Verification items for the finished model (mm, model axes). Face numbers are marked on the shaded views. A direction names the side the tool comes from. Coordinates: 2 decimals unless noted, no trailing zeros. Write each loop counter-clockwise with the first axis right and the second up, starting at its lowest first coordinate (ties: lowest second). Pieces come first, ordered by that corner, then holes. Notation, with made-up numbers: (31.5, 89.5) -> (81.5, 89.5) arc R17 ccw to (81.5, 100.5) -> close; hole circle Ø8 at (27, 55.5). An arc over 180 degrees is marked (long way). Use a Markdown table: item, result. Add a question column.
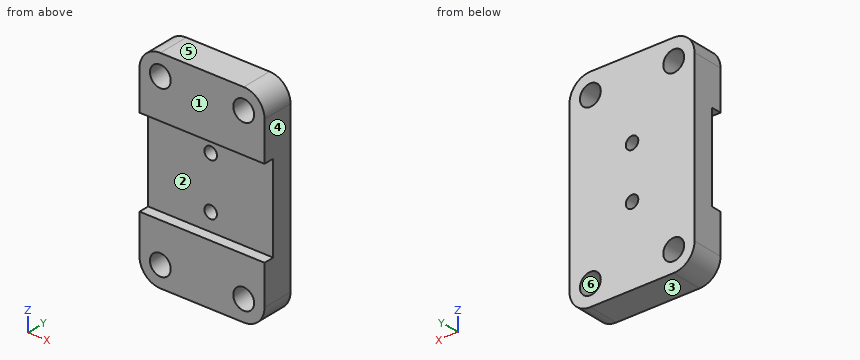
Autodesk Inventor part; units mm, degrees
ref_plane "YZ Plane" through (0, 0, 0) normal (1, 0, 0) x (0, 1, 0)
ref_plane "XZ Plane" through (0, 0, 0) normal (0, 1, 0) x (-1, 0, 0)
ref_plane "XY Plane" through (0, 0, 0) normal (0, 0, 1) x (1, 0, 0)
sketch "Sketch1" plane through (0, 0, 0) normal (0, 1, 0) x (-1, 0, 0)
  line L0 (30, 50) -> (-30, 50)
  line L1 (-30, 50) -> (-30, -50)
  line L2 (-30, -50) -> (30, -50)
  line L3 (30, -50) -> (30, 50)
  line L4 (30, 0) -> (-30, 0) construction
  line L5 (0, 50) -> (0, -50) construction
  circle A0 centre (20, 40) radius 5
  circle A1 centre (-20, 40) radius 5
  circle A2 centre (20, -40) radius 5
  circle A3 centre (-20, -40) radius 5
  circle A4 centre (0, -12.5) radius 3
  circle A5 centre (0, 12.5) radius 3
  point P0 (0, 0)
  point P1 (0, 0)
  dimension "d0" = 60
  dimension "d1" = 100
  dimension "d2" = 10
  dimension "d3" = 40
  dimension "d4" = 80
  dimension "d14" = 6
  dimension "d15" = 25
extrude "Extrusion1" add sketch "Sketch1" along normal blind 15
fillet "Fillet1" radius 10 4 edges at (30, 7.5, 50) (30, 7.5, -50) (-30, 7.5, 50) (-30, 7.5, -50)
sketch "Sketch2" plane through (30, 0, 40) normal (1, 0, 0) x (0, 0, -1)
  line L0 (80, 15) -> (80, 0) construction
  line L1 (0, 15) -> (80, 15) construction
  line L2 (0, 0) -> (0, 15) construction
  line L3 (0, 0) -> (80, 0) construction
  line L4 (19, 5) -> (61, 5)
  line L5 (61, 5) -> (61, 0)
  line L6 (61, 0) -> (19, 0)
  line L7 (19, 0) -> (19, 5)
  line L8 (40, 0) -> (40, 15) construction
  line L9 (0, 15) -> (80, 15) construction
  point P0 (40, 5)
  dimension "d9" = 42
  dimension "d10" = 5
extrude "Extrusion2" cut sketch "Sketch2" against normal through all
properties part number "base_obj1"
1) Release check for a two-part mould opening along Z. For the marked faces 3, 4, 5 and 6 record: released by +Z, released by -Z, zero draft, split by the parting line, or undercut.
2) Cross-section at A-A on y = 2.25. Record the boundary of the cut face in (x, z), then the cut area to 3 significant figures.
3) Cross-section at D-D on z = -36. Record the boundary of the cut face in (x, y).
4) Thickness scan on L1, parallel to Z at x = -20, y = 8.5; L2, parallel to Z at x = 20, y = 4.5; L3, parallel to Z at x = 0, y = 11.75. Record the ranges inside material, lowest first.
5) Cross-section at C-C on x = -12. Record the boundary of the cut face in (y, z), then the cut area to 3 significant figures.
6) Set-up check for the marked faces 1 and 2: record each of +Z, -Z, +X, -X, +Y, -Y from which the full face is reachable in a straight line by a thin tool's end or side.
7) Cross-section at B-B on z = -12.5. Record the boundary of the cut face in (x, y), then the cut area to 3 significant figures.
8) Gauge pin test, flat end, axial feed: pin 1 (1.5 mm diameter, centred on x = -19, z = 19.5, fed in from -Y). Record the tip position at first contact, or that the pin passes through.
Returned:
| question | item | result |
|---|---|---|
| 1 | face 3 | released by -Z |
| 1 | face 4 | zero draft |
| 1 | face 5 | released by +Z |
| 1 | face 6 | undercut |
| 2 | outline | (-30, -40) arc R10 ccw to (-20, -50) -> (20, -50) arc R10 ccw to (30, -40) -> (30, -21) -> (-30, -21) -> close; (-30, 21) -> (30, 21) -> (30, 40) arc R10 ccw to (20, 50) -> (-20, 50) arc R10 ccw to (-30, 40) -> close; hole circle Ø10 at (-20, -40); hole circle Ø10 at (-20, 40); hole circle Ø10 at (20, -40); hole circle Ø10 at (20, 40) |
| 2 | area | 3,080 mm² |
| 3 | outline | (-30, 0) -> (-23, 0) -> (-23, 15) -> (-30, 15) -> close; (-17, 0) -> (17, 0) -> (17, 15) -> (-17, 15) -> close; (23, 0) -> (30, 0) -> (30, 15) -> (23, 15) -> close |
| 4 | L1 | z = -50 to -45, -35 to 35, 45 to 50 |
| 4 | L2 | z = -50 to -45, -35 to -21, 21 to 35, 45 to 50 |
| 4 | L3 | z = -50 to -15.5, -9.5 to 9.5, 15.5 to 50 |
| 5 | outline | (0, -50) -> (15, -50) -> (15, 50) -> (0, 50) -> (0, 21) -> (5, 21) -> (5, -21) -> (0, -21) -> close |
| 5 | area | 1,290 mm² |
| 6 | face 1 | +Z, -Z, +X, -X, -Y |
| 6 | face 2 | +X, -X, -Y |
| 7 | outline | (-30, 5) -> (-3, 5) -> (-3, 15) -> (-30, 15) -> close; (3, 5) -> (30, 5) -> (30, 15) -> (3, 15) -> close |
| 7 | area | 540 mm² |
| 8 | pin 1 | stops at y = 5 |
